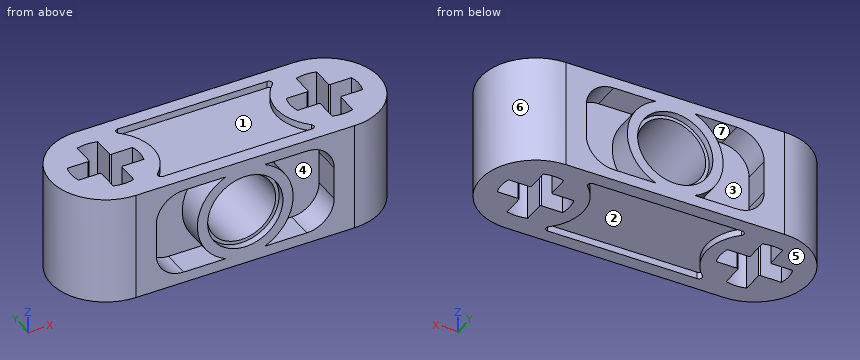
from build123d import *

# Parameters (mm, degrees)
EXTRUIR1_DEPTH         = 4
CROQUIS2_R             = 2.5
CORTAR_EXTRUIR1_DEPTH  = 9
CROQUIS3_R             = 2.75
CORTAR_EXTRUIR2_DEPTH  = 0.5
CORTAR_EXTRUIR3_DEPTH  = 2
SIMETR_A3_COPY_1_DEPTH = 2
REDONDEO1_R            = 2
CORTAR_EXTRUIR4_DEPTH  = 0.5


with BuildPart() as part:
    # Croquis1 → Extruir1 (new body, symmetric)
    with BuildSketch(Plane.XY):
        with BuildLine():
            Line((-8, 4), (8, 4))
            ThreePointArc((8, 4), (12, 0), (8, -4))
            Line((8, -4), (-8, -4))
            ThreePointArc((-8, -4), (-12, 0), (-8, 4))
        make_face()
        with BuildLine():
            Line((10.384848004, -0.75), (8.85, -0.75))
            ThreePointArc((8.85, -0.75), (8.779289322, -0.779289322), (8.75, -0.85))
            Line((8.75, -0.85), (8.75, -2.384848004))
            ThreePointArc((8.75, -2.384848004), (8, -2.5), (7.25, -2.384848004))
            Line((7.25, -2.384848004), (7.25, -0.85))
            ThreePointArc((7.25, -0.85), (7.220710678, -0.779289322), (7.15, -0.75))
            Line((7.15, -0.75), (5.615151996, -0.75))
            ThreePointArc((5.615151996, -0.75), (5.5, 0), (5.615151996, 0.75))
            Line((5.615151996, 0.75), (7.15, 0.75))
            ThreePointArc((7.15, 0.75), (7.220710678, 0.779289322), (7.25, 0.85))
            Line((7.25, 0.85), (7.25, 2.384848004))
            ThreePointArc((7.25, 2.384848004), (8, 2.5), (8.75, 2.384848004))
            Line((8.75, 2.384848004), (8.75, 0.85))
            ThreePointArc((8.75, 0.85), (8.779289322, 0.779289322), (8.85, 0.75))
            Line((8.85, 0.75), (10.384848004, 0.75))
            ThreePointArc((10.384848004, 0.75), (10.5, 0), (10.384848004, -0.75))
        make_face(mode=Mode.SUBTRACT)
        with BuildLine():
            Line((-10.384848004, 0.75), (-8.85, 0.75))
            ThreePointArc((-8.85, 0.75), (-8.779289322, 0.779289322), (-8.75, 0.85))
            Line((-8.75, 0.85), (-8.75, 2.384848004))
            ThreePointArc((-8.75, 2.384848004), (-8, 2.5), (-7.25, 2.384848004))
            Line((-7.25, 2.384848004), (-7.25, 0.85))
            ThreePointArc((-7.25, 0.85), (-7.220710678, 0.779289322), (-7.15, 0.75))
            Line((-7.15, 0.75), (-5.615151996, 0.75))
            ThreePointArc((-5.615151996, 0.75), (-5.5, 0), (-5.615151996, -0.75))
            Line((-5.615151996, -0.75), (-7.15, -0.75))
            ThreePointArc((-7.15, -0.75), (-7.220710678, -0.779289322), (-7.25, -0.85))
            Line((-7.25, -0.85), (-7.25, -2.384848004))
            ThreePointArc((-7.25, -2.384848004), (-8, -2.5), (-8.75, -2.384848004))
            Line((-8.75, -2.384848004), (-8.75, -0.85))
            ThreePointArc((-8.75, -0.85), (-8.779289322, -0.779289322), (-8.85, -0.75))
            Line((-8.85, -0.75), (-10.384848004, -0.75))
            ThreePointArc((-10.384848004, -0.75), (-10.5, 0), (-10.384848004, 0.75))
        make_face(mode=Mode.SUBTRACT)
    extrude(amount=EXTRUIR1_DEPTH, both=True)

    # Croquis2 → Cortar-Extruir1 (cut, through all)
    with BuildSketch(Plane(origin=(0, 4, 0), x_dir=(-1, 0, 0), z_dir=(0, 1, 0))):
        Circle(CROQUIS2_R)
    extrude(amount=-CORTAR_EXTRUIR1_DEPTH, mode=Mode.SUBTRACT)

    # Croquis3 → Cortar-Extruir2 (cut)
    with BuildSketch(Plane(origin=(0, 4, 0), x_dir=(-1, 0, 0), z_dir=(0, 1, 0))):
        Circle(CROQUIS3_R)
    cortar_extruir2 = extrude(amount=-CORTAR_EXTRUIR2_DEPTH, mode=Mode.SUBTRACT)

    # Simetría1: Cortar-Extruir2 across plane
    add(cortar_extruir2.mirror(Plane.ZX), mode=Mode.SUBTRACT)

    # Croquis4 → Cortar-Extruir3 (cut)
    with BuildSketch(Plane(origin=(0, 4, 0), x_dir=(-1, 0, 0), z_dir=(0, 1, 0))):
        with BuildLine():
            Line((-1.417744688, -3.2), (-6.5, -3.2))
            Line((-6.5, -3.2), (-6.5, 3.2))
            Line((-6.5, 3.2), (-1.417744688, 3.2))
            ThreePointArc((-1.417744688, 3.2), (-3.5, 0), (-1.417744688, -3.2))
        make_face()
    cortar_extruir3 = extrude(amount=-CORTAR_EXTRUIR3_DEPTH, mode=Mode.SUBTRACT)

    # Simetría2: Cortar-Extruir3 across plane
    add(cortar_extruir3.mirror(Plane(origin=(0, 0, 0), x_dir=(0, 0, 1), z_dir=(1, 0, 0))), mode=Mode.SUBTRACT)

    # Simetría3: Cortar-Extruir3 across plane
    add(cortar_extruir3.mirror(Plane.ZX), mode=Mode.SUBTRACT)

    # Simetría3 copy 1 sketch → Simetría3 copy 1 (cut)
    with BuildSketch(Plane.XZ.offset(4)):
        with BuildLine():
            Line((-1.417744688, -3.2), (-6.5, -3.2))
            Line((-6.5, -3.2), (-6.5, 3.2))
            Line((-6.5, 3.2), (-1.417744688, 3.2))
            ThreePointArc((-1.417744688, 3.2), (-3.5, 0), (-1.417744688, -3.2))
        make_face()
    extrude(amount=-SIMETR_A3_COPY_1_DEPTH, mode=Mode.SUBTRACT)

    # Redondeo1
    redondeo1_edges = [part.edges().sort_by_distance(p)[0] for p in [
        (6.5, 3, -3.2),
        (6.5, 3, 3.2),
        (-6.5, 3, 3.2),
        (-6.5, 3, -3.2),
        (-6.5, -3, -3.2),
        (-6.5, -3, 3.2),
        (6.5, -3, 3.2),
        (6.5, -3, -3.2),
    ]]
    fillet(redondeo1_edges, radius=REDONDEO1_R)

    # Croquis5 → Cortar-Extruir4 (cut)
    with BuildSketch(Plane.XY.offset(4)):
        with BuildLine():
            Line((-5.450490243, 3), (5.450490243, 3))
            ThreePointArc((5.450490243, 3), (5.683227577, 2.841287093), (5.62045756, 2.566666667))
            ThreePointArc((5.62045756, 2.566666667), (4.5, 0), (5.62045756, -2.566666667))
            ThreePointArc((5.62045756, -2.566666667), (5.683227577, -2.841287093), (5.450490243, -3))
            Line((5.450490243, -3), (-5.450490243, -3))
            ThreePointArc((-5.450490243, -3), (-5.683227577, -2.841287093), (-5.62045756, -2.566666667))
            ThreePointArc((-5.62045756, -2.566666667), (-4.5, 0), (-5.62045756, 2.566666667))
            ThreePointArc((-5.62045756, 2.566666667), (-5.683227577, 2.841287093), (-5.450490243, 3))
        make_face()
    cortar_extruir4 = extrude(amount=-CORTAR_EXTRUIR4_DEPTH, mode=Mode.SUBTRACT)

    # Simetría4: Cortar-Extruir4 across plane
    add(cortar_extruir4.mirror(Plane.XY), mode=Mode.SUBTRACT)


solid = part.part
Read the model definition and answer for the solid it produces. Units are mm, in the model's axes. Face numbers are marked on the shaded views. A direction names the side the tool comes from. Coordinates: 2 decimals unless noted, no trailing zeros. Order: outer loops, then holes, each group sorted by start corner. A loop starts at its lowest first (then second) coordinate and runs counter-clockwise, first axis right, second up. Notation, with made-up numbers: (85.25, -9) - (97.25, -9) arc R14 ccw to (97.25, 5) - close; hole circle Ø3 at (52.25, 70.25). An arc over 180 degrees is marked (long way). Use one line per item in the form item = value.
(1) Which of the six approach directions +Z, -Z, +X, -X, +Y, -Y give full straight-line access (tool end or side, diameter ignored) to the marked faces 1, 2, 3 and 4?
Computed values:
face_1 = +Z
face_2 = -Z
face_3 = +Y
face_4 = -Y
(2) Straight lines are drawn through the part: L1, parallel to Z at x = 0, y = 3.65; L2, parallel to X at y = -1.25, z = -1.75; L3, parallel to Z at x = 0, y = -1.75. For each, find the intervals that lie inside material, in ascending order.
Computed values:
L1 = -4 to -2.75, 2.75 to 4
L2 = -11.8 to -8.75, -7.25 to -1.79, 1.79 to 7.25, 8.75 to 11.8
L3 = -3.5 to -2.5, 2.5 to 3.5
(3) For a pull along Z with two mould halves and no side action, classify the marked faces 5, 6 and 7 as pulls with the +Z half, pulls with the -Z half, needs draft (parallel to the pull), parting line crosses it, or undercut.
Computed values:
face_5 = pulls with the -Z half
face_6 = needs draft
face_7 = undercut
(4) Section A-A, the plane x = 0 is taken. Give the vertices of the cut face in (y, z).
Computed values:
outline = (-4, -4) - (-3, -4) - (-3, -3.5) - (3, -3.5) - (3, -4) - (4, -4) - (4, -2.75) - (3.5, -2.75) - (3.5, -2.5) - (-3.5, -2.5) - (-3.5, -2.75) - (-4, -2.75) - close; (-4, 2.75) - (-3.5, 2.75) - (-3.5, 2.5) - (3.5, 2.5) - (3.5, 2.75) - (4, 2.75) - (4, 4) - (3, 4) - (3, 3.5) - (-3, 3.5) - (-3, 4) - (-4, 4) - close
(5) Section C-C, the plane x = -3.75 is taken. Give the vertices of the cut face in (y, z), then the cut area to 3 significant figures.
Computed values:
outline = (-4, -4) - (-3, -4) - (-3, -3.5) - (3, -3.5) - (3, -4) - (4, -4) - (4, -3.2) - (2, -3.2) - (2, 3.2) - (4, 3.2) - (4, 4) - (3, 4) - (3, 3.5) - (-3, 3.5) - (-3, 4) - (-4, 4) - (-4, 3.2) - (-2, 3.2) - (-2, -3.2) - (-4, -3.2) - close
area = 32.4 mm²
(6) Section D-D, the plane z = -1.5 is taken. Give the number of separate pieces and of enclosed holes in the cut face, then the cut area to 3 significant figures.
Computed values:
separate_pieces = 2
enclosed_holes = 2
area = 94.1 mm²
(7) Section B-B, the plane y = 0.5 is taken. Give the vertices of the cut face in (x, z), then the cut area to 3 significant figures.
Computed values:
outline = (-11.97, -4) - (-10.45, -4) - (-10.45, 4) - (-11.97, 4) - close; (-5.55, -4) - (-4.54, -4) - (-4.54, -3.5) - (4.54, -3.5) - (4.54, -4) - (5.55, -4) - (5.55, 4) - (4.54, 4) - (4.54, 3.5) - (-4.54, 3.5) - (-4.54, 4) - (-5.55, 4) - close; (10.45, -4) - (11.97, -4) - (11.97, 4) - (10.45, 4) - close; hole circle Ø5 at (0, 0)
area = 84.4 mm²
(8) Given pin 1 Ø1.7 at (y, z) = (1.5, 1) entering from -X; pin 2 Ø1.7 at (x, z) = (-10, 1) entering from +Y; pin 3 Ø0.5 at (y, z) = (2, 0) entering from -X; pin 4 Ø2 at (x, z) = (-3.5, -2) entering from +Y, each flat-ended and moving along its own axis, determine where each tip first touches the part or whether it passes through.
Computed values:
pin_1 = -11.95
pin_2 = 3.83
pin_3 = -11.6
pin_4 = 4
